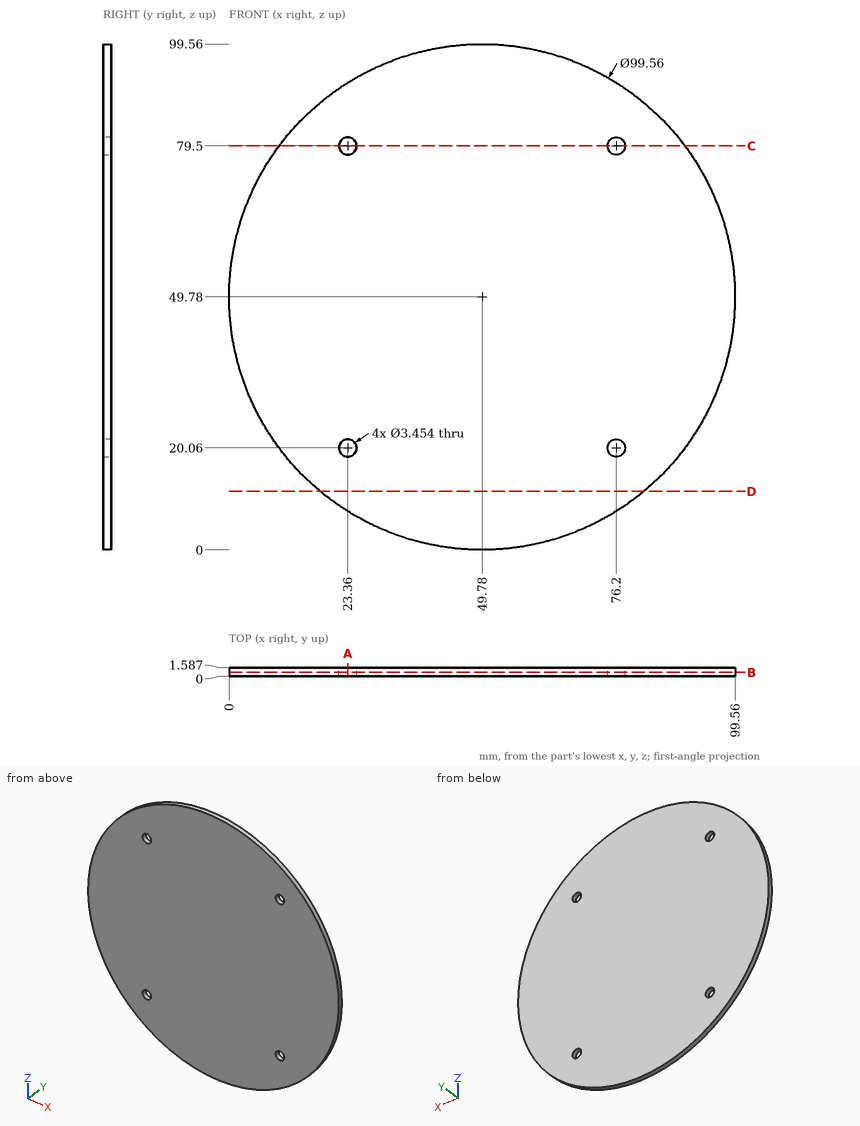
Geometry check sheet. Reference: drawing and pictorial views, mm from the part's lowest x, y, z. Give positions to 0.01 mm unless a question says otherwise; leave off trailing zeros. Loops run counter-clockwise (first coordinate to the right, second up) from the corner with the lowest first, then second, coordinate; pieces in that order, holes last. Notation, with made-up numbers: (30.25, -3.5) -> (39.25, -3.5) arc R18 ccw to (39.25, 13.5) -> close; hole circle Ø5 at (-12, -5.5). An arc over 180 degrees is marked (long way). Answer in a Markdown table with one row per item. Add a question column.
1) Cross-section at A-A on x = 23.36. Record the boundary of the cut face in (y, z).
2) Cross-section at D-D on z = 11.5. Record the boundary of the cut face in (x, y).
3) Gauge pin test, flat end, axial feed: P1, Ø2, axis at x = 23.36, z = 79.5, coming from the +Y side (1 decimal). Record the tip position at first contact, or that the pin passes through.
4) Cross-section at B-B on y = 0.7. Record the boundary of the cut face in (x, z) (1 decimal), and give its area (3 significant figures).
5) Material ranges on probe 1 along X at (y, z) = (0.65, 20.06) (1 decimal); probe 2 along X at (y, z) = (1.5, 19.5) (1 decimal); probe 3 along Z at (x, y) = (76.2, 0.9) (1 decimal), recorded low to high. Write a range as from..to.
6) Cross-section at C-C on z = 79.5. Record the boundary of the cut face in (x, y) (1 decimal).
Outcome:
| question | item | result |
|---|---|---|
| 1 | outline | (0, 7.59) -> (1.59, 7.59) -> (1.59, 18.33) -> (0, 18.33) -> close; (0, 21.79) -> (1.59, 21.79) -> (1.59, 77.77) -> (0, 77.77) -> close; (0, 81.23) -> (1.59, 81.23) -> (1.59, 91.97) -> (0, 91.97) -> close |
| 2 | outline | (17.96, 0) -> (81.6, 0) -> (81.6, 1.59) -> (17.96, 1.59) -> close |
| 3 | P1 | passes through |
| 4 | outline | circle Ø99.6 at (49.8, 49.8); hole circle Ø3.5 at (23.4, 20.1); hole circle Ø3.5 at (23.4, 79.5); hole circle Ø3.5 at (76.2, 20.1); hole circle Ø3.5 at (76.2, 79.5) |
| 4 | area | 7,750 mm^2 |
| 5 | probe 1 | x = 9.8..21.6, 25.1..74.5, 77.9..89.7 |
| 5 | probe 2 | x = 10.3..21.7, 25..74.6, 77.8..89.3 |
| 5 | probe 3 | z = 7.6..18.3, 21.8..77.8, 81.2..92 |
| 6 | outline | (9.8, 0) -> (21.6, 0) -> (21.6, 1.6) -> (9.8, 1.6) -> close; (25.1, 0) -> (74.5, 0) -> (74.5, 1.6) -> (25.1, 1.6) -> close; (77.9, 0) -> (89.7, 0) -> (89.7, 1.6) -> (77.9, 1.6) -> close |
